Study the drawing (mm; zero at the part's minimum x, y, z) and answer. A direction names the side the tool comes from. Coordinates: 2 decimals unless noted, no trailing zeros. Order: outer loops, then holes, each group sorted by start corner. A loop starts at its lowest first (then second) coordinate and runs counter-clockwise, first axis right, second up. Notation, with made-up numbers: M 43,86 L 56,86 A21 ccw 56,111 Z; hole C -40,-11.5 d7. An arc over 180 degrees is marked long. Use a Markdown table: item, result. Add a question column.
1) Find section A-A on x = 5. Write down the section's boundary in (y, z) (3 decimals), plus the area to 3 significant figures.
2) Find section B-B on y = 151. Write down the section's boundary in (x, z), plus the area to 3 significant figures.
3) Find section C-C on z = 4.5. Write down the section's boundary in (x, y).
4) Each of these flat-tipped pins is pushed along its axis until it touches: pin 1 Ø4 at (x, y) = (5, 66) entering from +Z; pin 2 Ø1.5 at (x, y) = (8, 85) entering from -Z; pin 3 Ø1 at (x, y) = (5.5, 120.5) entering from -Z. Where does it stop, or does it pass through?
5) Find the intervals of material crossed by probe 1 along Z at (x, y) = (5.75, 206) (3 decimals); probe 2 along Y at (x, z) = (5, 22.5); probe 3 along X at (y, z) = (146, 22.1), in increasing order. Write a range as [from, to].
6) For the marked faces 1, 2, 3 and 4, determine the directions among +Z, -Z, +X, -X, +Y, -Y from which every point of the face is accessible in a straight line to the end or side of a thin tool.
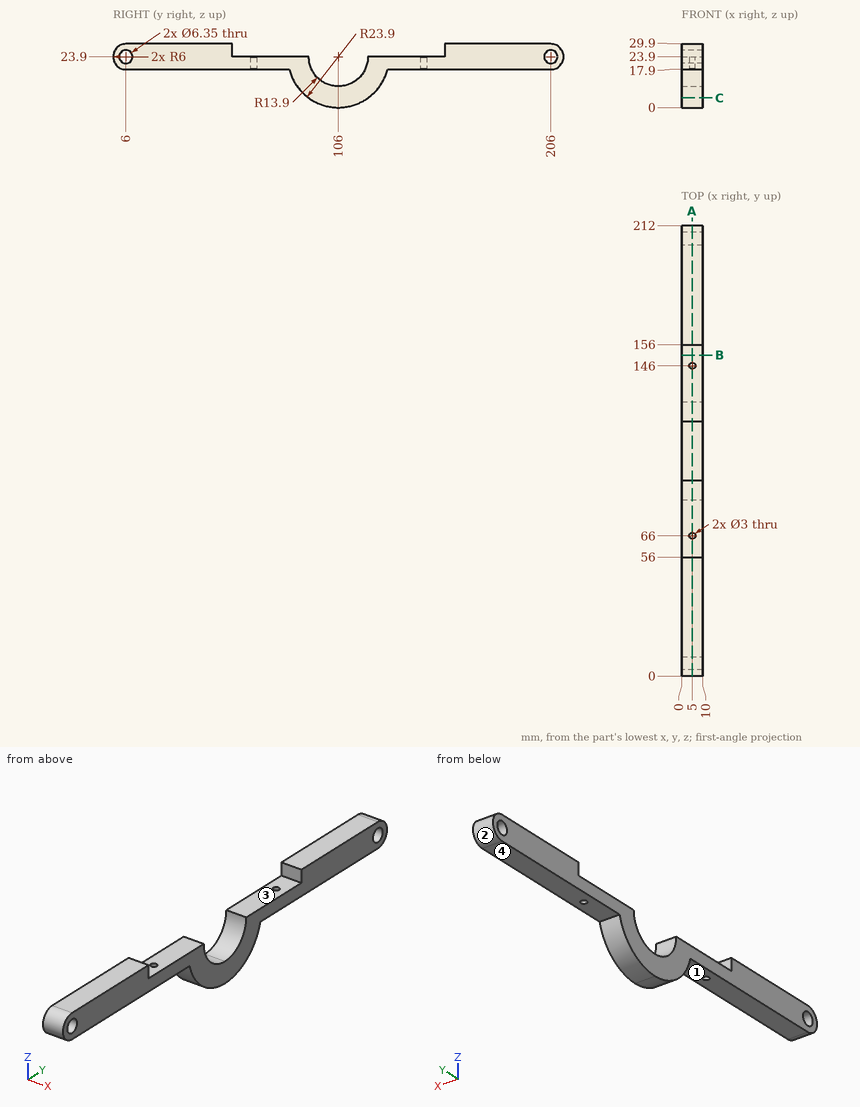
Check result:
| question | item | result |
|---|---|---|
| 1 | outline | M 6,17.9 L 64.5,17.9 L 64.5,23.9 L 56,23.9 L 56,29.9 L 6,29.9 A6 ccw Z; M 67.5,17.9 L 82.865,17.9 A23.9 ccw 106,0 A23.9 ccw 129.135,17.9 L 144.5,17.9 L 144.5,23.9 L 119.9,23.9 A13.9 cw 106,10 A13.9 cw 92.1,23.9 L 67.5,23.9 Z; M 147.5,17.9 L 206,17.9 A6 ccw 206,29.9 L 156,29.9 L 156,23.9 L 147.5,23.9 Z; hole C 6,23.9 d6.35; hole C 206,23.9 d6.35 |
| 1 | area | 2,120 mm2 |
| 2 | outline | M 0,17.9 L 10,17.9 L 10,23.9 L 0,23.9 Z |
| 2 | area | 60.0 mm2 |
| 3 | outline | M 0,92.04 L 10,92.04 L 10,119.96 L 0,119.96 Z |
| 4 | pin 1 | stops at z = 23.9 |
| 4 | pin 2 | stops at z = 11.21 |
| 4 | pin 3 | stops at z = 4.53 |
| 5 | probe 1 | z = [17.9, 20.725], [27.075, 29.9] |
| 5 | probe 2 | y = [0.17, 3.15], [8.85, 64.5], [67.5, 92.17], [119.83, 144.5], [147.5, 203.15], [208.85, 211.83] |
| 5 | probe 3 | x = [0, 3.5], [6.5, 10] |
| 6 | face 1 | -Z, +X, -X, -Y |
| 6 | face 2 | +X, -X, +Y |
| 6 | face 3 | +Z, +X, -X |
| 6 | face 4 | -Z, +X, -X, +Y |
